Answer from the drawing. Dimensions are ordinates in mm from the lowest x, y and z of the part. A direction names the side the tool comes from. Coordinates: 2 decimals unless noted, no trailing zeros. Answer in a Markdown table with one row per item.
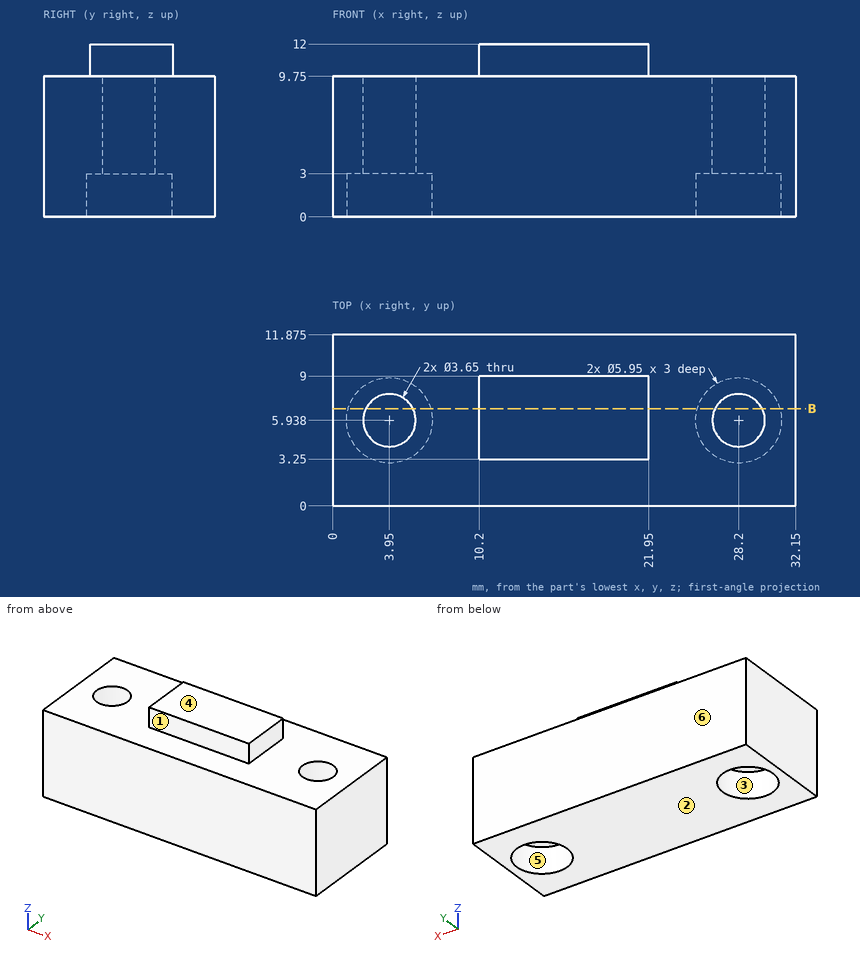
Q1. Given pin 1 (3 mm diameter, centred on x = 4.5, y = 7, fed in from -Z); pin 2 (4 mm diameter, centred on x = 28.2, y = 5.94, fed in from +Z); pin 3 (0.7 mm diameter, centred on y = 6, z = 11, fed in from -X), each flat-ended and moving along its own axis, determine where each tip first touches the part or whether it passes through.
Outcome:
| item | result |
|---|---|
| pin 1 | z = 3 |
| pin 2 | z = 9.75 |
| pin 3 | x = 10.2 |
Q2. The part is cut by section B-B (y = 6.75). Give the number of separate pieces and of enclosed holes in the cut face.
Outcome:
| item | result |
|---|---|
| separate pieces | 3 |
| enclosed holes | 0 |
Q3. For a pull along Y with two mould halves and no side action, classify the marked faces 3, 4, 5 and 6 as pulls with the +Y half, pulls with the -Y half, needs draft (parallel to the pull), parting line crosses it, or undercut.
Outcome:
| item | result |
|---|---|
| face 3 | undercut |
| face 4 | needs draft |
| face 5 | undercut |
| face 6 | pulls with the +Y half |
Q4. For the marked faces 1 and 2, determine the directions among +Z, -Z, +X, -X, +Y, -Y from which every point of the face is accessible in a straight line to the end or side of a thin tool.
Outcome:
| item | result |
|---|---|
| face 1 | +Z, +X, -X, -Y |
| face 2 | -Z, +X, -X, +Y, -Y |
Q5. Consider line 1 (X direction, y = 5.25, z = 8.75); line 2 (Y direction, x = 28.2, z = 7.5) (1 decimal); line 3 (X direction, y = 5.5, z = 2.5). Determine where each line is inside the solid, lowest interval first.
Outcome:
| item | result |
|---|---|
| line 1 | 0 to 2.26, 5.64 to 26.51, 29.89 to 32.15 |
| line 2 | 0 to 4.1, 7.8 to 11.9 |
| line 3 | 0 to 1.01, 6.89 to 25.26, 31.14 to 32.15 |
